from build123d import *

# Parameters (mm, degrees)
SKETCH_W     = 89
SKETCH_H     = 42
PAD_DEPTH    = 2
SKETCH001_W  = 50
SKETCH001_H  = 30
PAD001_DEPTH = 8
SKETCH002_R  = 1.5
POCKET_DEPTH = 2
SKETCH003_W  = 6
SKETCH003_H  = 9
PAD002_DEPTH = 3
SKETCH005_W  = 78
SKETCH005_H  = 42
PAD003_DEPTH = 22


with BuildPart() as part:
    # Sketch → Pad (new body)
    with BuildSketch(Plane.XY):
        Rectangle(SKETCH_W, SKETCH_H)
    extrude(amount=PAD_DEPTH)

    # Sketch001 (on Face6 of Pad) → Pad001 (join)
    with BuildSketch(Plane.XY.offset(2)):
        Rectangle(SKETCH001_W, SKETCH001_H)
    extrude(amount=PAD001_DEPTH)

    # Sketch002 (on Face5 of Pad001) → Pocket (cut)
    with BuildSketch(Plane.XY.offset(2)):
        with Locations((-42, 18.5)):
            Circle(SKETCH002_R)
        with Locations((42, 18.5)):
            Circle(SKETCH002_R)
        with Locations((-42, -18.5)):
            Circle(SKETCH002_R)
        with Locations((42, -18.5)):
            Circle(SKETCH002_R)
    extrude(amount=-POCKET_DEPTH, mode=Mode.SUBTRACT)

    # Sketch003 (on Face5 of Pocket) → Pad002 (join)
    with BuildSketch(Plane.XY.offset(2)):
        with Locations((-43.5, 0)):
            Rectangle(SKETCH003_W, SKETCH003_H)
    extrude(amount=PAD002_DEPTH)

    # Sketch005 → Pad003 (join)
    with BuildSketch(Plane.XY):
        Rectangle(SKETCH005_W, SKETCH005_H)
    extrude(amount=-PAD003_DEPTH)


with BuildPart() as part_1:
    # Body placement: moved
    add(part.part.moved(Location((3, 0, 24))))


solid = part_1.part
Could you check a few things on this model? Use its own coordinates, in mm. A direction names the side the tool comes from. Coordinates: 2 decimals unless noted, no trailing zeros. Write each loop counter-clockwise with the first axis right and the second up, starting at its lowest first coordinate (ties: lowest second). Pieces come first, ordered by that corner, then holes. Notation, with made-up numbers: M -3.5,-22 L 9.5,-22 A5 ccw 9.5,-17 Z; hole C 89.25,-27 d11. An arc over 180 degrees is marked long. One line per question, with ' | ' between items.
1) Imagine slicing it at D-D, the plane y = 0. Write out the boundary of the cut face in (x, z), and give its area (3 significant figures).
Checks:
outline: M -43.5,26 L -41.5,26 L -41.5,24 L -36,24 L -36,2 L 42,2 L 42,24 L 47.5,24 L 47.5,26 L 28,26 L 28,34 L -22,34 L -22,26 L -37.5,26 L -37.5,29 L -43.5,29 Z | area: 2,310 mm²
2) I need wall thicknesses on probe 1 along Y at (x, z) = (45, 24.95); probe 2 along X at (y, z) = (18, 25); probe 3 along Z at (x, y) = (4, 18). Which ranges of each line are inside material? Lowest first, please. Write a range as [from, to].
Checks:
probe 1: [-21, -20], [-17, 17], [20, 21] | probe 2: [-41.5, -40.41], [-37.59, 43.59], [46.41, 47.5] | probe 3: [2, 26]
3) Imagine slicing it at C-C, the plane x = 5.5. Write out the boundary of the cut face in (y, z), and give its area (3 significant figures).
Checks:
outline: M -21,2 L 21,2 L 21,26 L 15,26 L 15,34 L -15,34 L -15,26 L -21,26 Z | area: 1,250 mm²
4) For faces 4 (the face through (3, 15, 30)), 5 (the face through (-37.5, 0, 27)), 6 (the face through (-39, 0, 24)), 7 (the face through (45, 0, 24)), 8 (the face through (-41, -4.5, 27)), which set-ups out of +Z, -Z, +X, -X, +Y, -Y let a thin tool reach every point of the face, with its end or its side?
Checks:
face 4: +Z, +X, -X, +Y | face 5: +Z, +Y, -Y | face 6: -Z, -X, +Y, -Y | face 7: -Z, +X, +Y, -Y | face 8: +Z, -X, -Y
5) Imagine slicing it at B-B, the plane x = -39. Write out the boundary of the cut face in (y, z), and give its area (3 significant figures).
Checks:
outline: M -21,24 L -20,24 L -20,26 L -21,26 Z; M -17,24 L 17,24 L 17,26 L 4.5,26 L 4.5,29 L -4.5,29 L -4.5,26 L -17,26 Z; M 20,24 L 21,24 L 21,26 L 20,26 Z | area: 99.0 mm²
6) If we mould it in two halves opening along Y, with no side actions, what happens to faces 1 (the face through (43.5, -18.43, 25.01)), 2 (the face through (-41, 4.5, 27)), 3 (the face through (2, 0, 2))? For each: released by +Y, released by -Y, zero draft, split by the parting line, or undercut.
Checks:
face 1: undercut | face 2: released by +Y | face 3: zero draft
7) Imagine slicing it at A-A, the plane y = 18.5. Write out the boundary of the cut face in (x, z).
Checks:
outline: M -41.5,24 L -40.5,24 L -40.5,26 L -41.5,26 Z; M -37.5,24 L -36,24 L -36,2 L 42,2 L 42,24 L 43.5,24 L 43.5,26 L -37.5,26 Z; M 46.5,24 L 47.5,24 L 47.5,26 L 46.5,26 Z
8) For pin 1 Ø2.5 at (y, z) = (0.5, 30.5) entering from +X; pin 2 Ø12 at (y, z) = (16.5, 11.5) entering from +X; pin 3 Ø1.6 at (x, y) = (44, -6.5) entering from -Z, each with a flat end and sliding along its axis, tell me the tip position at first contact or that it passes through.
Checks:
pin 1: x = 28 | pin 2: x = 42 | pin 3: z = 24
